```python
from build123d import *

# Parameters (mm, degrees)
SKETCH1_R            = 8.509
BOSS_EXTRUDE1_DEPTH  = 3.81
SKETCH3_W            = 7.9375
SKETCH3_H            = 5.08
CUT_EXTRUDE2_DEPTH   = 3.81
M2_CLEARANCE_HOLE1_D = 2.4
FILLET1_R            = 1.5875
CHAMFER1_SIZE        = 0.75


with BuildPart() as part:
    # Sketch1 → Boss-Extrude1 (new body)
    with BuildSketch(Plane.XY):
        Circle(SKETCH1_R)
    extrude(amount=BOSS_EXTRUDE1_DEPTH)

    # Sketch3 → Cut-Extrude2 (cut)
    with BuildSketch(Plane.XY.offset(3.81)):
        Rectangle(SKETCH3_W, SKETCH3_H)
    extrude(amount=-CUT_EXTRUDE2_DEPTH, mode=Mode.SUBTRACT)

    # M2 Clearance Hole1 (through all)
    with Locations(Plane.XY.offset(3.81)):
        with Locations((-6.223, 0), (3.1115, 5.389276088), (3.1115, -5.389276088)):
            Hole(M2_CLEARANCE_HOLE1_D / 2)

    # Fillet1
    fillet1_edges = [part.edges().sort_by_distance(p)[0] for p in [
        (3.96875, 2.54, 1.905),
        (3.96875, -2.54, 1.905),
        (-3.96875, -2.54, 1.905),
        (-3.96875, 2.54, 1.905),
    ]]
    fillet(fillet1_edges, radius=FILLET1_R)

    # Chamfer1
    chamfer1_edges = [part.edges().sort_by_distance(p)[0] for p in [
        (4.3115, -5.389276088, 3.81),
        (4.3115, 5.389276088, 3.81),
        (-5.023, 0, 3.81),
    ]]
    chamfer(chamfer1_edges, length=CHAMFER1_SIZE)


solid = part.part
```
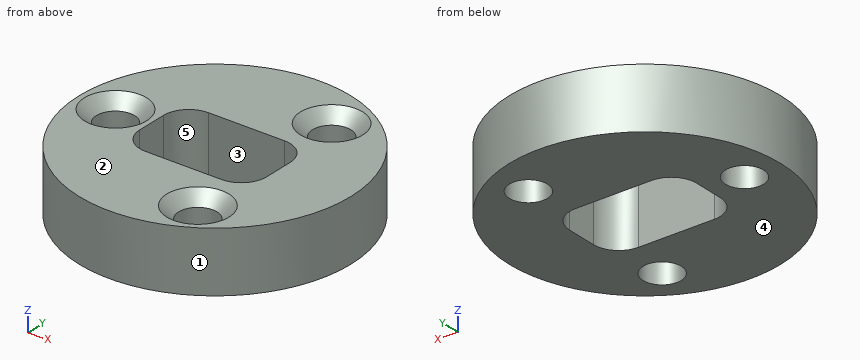
Build history of the part. All positions in model axes, mm. Face numbers are marked on the shaded views. A direction names the side the tool comes from. Coordinates: 2 decimals unless noted, no trailing zeros. Order: outer loops, then holes, each group sorted by start corner. A loop starts at its lowest first (then second) coordinate and runs counter-clockwise, first axis right, second up. Notation, with made-up numbers: M 33,31.25 L 41,31.25 A19 ccw 41,36.25 Z; hole C 7,-28 d4. An arc over 180 degrees is marked long. One line per question, with ' | ' between items. Start each with the question number.
1. Wall check: line 1 along Y through (x, z) = (2.5, 2); line 2 along Y through (x, z) = (3, 0.65); line 3 along X through (y, z) = (-1.25, 3.35). Give the ranges that are in metal, low to high. Write a range as [from, to].
2. Mould opens along X. For the marked faces 1, 2 and 3 say: +X half, -X half, draft (parallel to the pull), parting line (faces both ways), or undercut.
3. Cut at D-D (x = -2.75). Write the cut outline in (y, z), plus the area to 3 significant figures.
4. Cut at A-A (x = 0). Write the cut outline in (y, z), plus the area to 3 significant figures.
5. Cut at C-C (z = 1.55). Write the cut outline in (x, y) (1 decimal), plus the area to 3 significant figures.
6. Cut at B-B (y = 0). Write the cut outline in (x, z).
7. Flat gauge pins, fed straight in: P1, Ø2, axis at y = 3, z = 2, coming from the -X side; P2, Ø1.5, axis at y = 2, z = 0.5, coming from the -X side; P3, Ø2, axis at x = -1.5, z = 3, coming from the +Y side. Where does each tip first touch, or does it go through?
8. Tool access for the marked faces 4 and 5: list every direction of +Z, -Z, +X, -X, +Y, -Y with a clear straight run to the whole face (end or side of a thin tool).
The answers:
1) line 1: y = [-8.13, -6.42], [-4.36, -2.54], [2.54, 4.36], [6.42, 8.13] | line 2: y = [-7.96, -6.58], [-4.19, -2.41], [2.41, 4.19], [6.58, 7.96] | line 3: x = [-8.42, -7.03], [-5.41, -3.94], [3.94, 8.42]
2) face 1: parting line | face 2: draft | face 3: undercut
3) outline: M -8.05,0 L -2.5,0 L -2.5,3.81 L -8.05,3.81 Z; M 2.5,0 L 8.05,0 L 8.05,3.81 L 2.5,3.81 Z | area: 42.3 mm2
4) outline: M -8.51,0 L -2.54,0 L -2.54,3.81 L -8.51,3.81 Z; M 2.54,0 L 8.51,0 L 8.51,3.81 L 2.54,3.81 Z | area: 45.5 mm2
5) outline: C 0,0 d17; hole C -6.2,0 d2.4; hole M -4,-1 A1.6 ccw -2.4,-2.5 L 2.4,-2.5 A1.6 ccw 4,-1 L 4,1 A1.6 ccw 2.4,2.5 L -2.4,2.5 A1.6 ccw -4,1 Z; hole C 3.1,-5.4 d2.4; hole C 3.1,5.4 d2.4 | area: 176 mm2
6) outline: M -8.51,0 L -7.42,0 L -7.42,3.06 L -8.17,3.81 L -8.51,3.81 Z; M -5.02,0 L -3.97,0 L -3.97,3.81 L -4.27,3.81 L -5.02,3.06 Z; M 3.97,0 L 8.51,0 L 8.51,3.81 L 3.97,3.81 Z
7) P1: stops at x = -8.27 | P2: stops at x = -8.42 | P3: stops at y = 8.49
8) face 4: -Z, +X, -X, +Y, -Y | face 5: +Z, -Z
